Design review of the part built by this model. Coordinates are the model's own, in mm. Face numbers are marked on the shaded views. A direction names the side the tool comes from. Round coordinates to 2 decimals unless told otherwise and drop trailing zeros. Loops run counter-clockwise (first coordinate to the right, second up) from the corner with the lowest first, then second, coordinate; pieces in that order, holes last. Notation, with made-up numbers: M 39,53 L 87,53 A24 ccw 87,82 Z; hole C 0,25.25 d10. An arc over 180 degrees is marked long. One line per item, written item: value. Start each with the question number.
Item 1: Clearance check with a flat-ended pin moving along its axis: pin 1 (1 mm diameter, centred on y = 3, z = -19, fed in from +X). State where the tip first meets the part, or that it passes through.
Item 2: We need section C-C (z = -10.75). Write out the cut boundary in (x, y).
Item 3: For the marked faces 1 and 2, list the 3-axis set-ups (+Z, -Z, +X, -X, +Y, -Y) from which the entire face can be reached by the end or side of a thin tool; tool diameter is ignored.
Item 4: Mouldability with a two-part tool opening along Z and no side actions: class the marked faces 3, 4 and 5 as released by +Z, released by -Z, zero draft, split by the parting line, or undercut.
Item 5: We need section A-A (y = 0.55). Write out the cut boundary in (x, z).
Item 6: We need section B-B (x = -27.5). Write out the cut boundary in (y, z).
Item 7: We need section D-D (x = -29). Write out the cut boundary in (y, z).
Item 8: For line 1 along Z through (x, y) = (-27.75, 1.95); line 2 along Z through (x, y) = (-27.5, 2.1); line 3 along X through (y, z) = (0.45, -19.5), list the stretches that pass through material, from the lowest coordinate up.
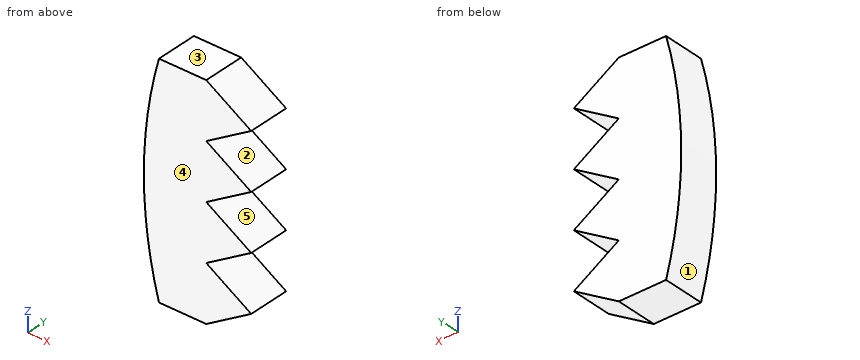
from build123d import *

# Parameters (mm, degrees)
BOSS_EXTRUDE1_DEPTH = 3.81


with BuildPart() as part:
    # Sketch1 → Boss-Extrude1 (new body)
    with BuildSketch(Plane(origin=(0, 0, 0), x_dir=(1, 0, 0), z_dir=(0, 1, 0))):
        with BuildLine():
            Line((-30.793742763, 27.560180372), (-26.69024718, 25.020180372))
            Line((-26.69024718, 25.020180372), (-30.793742763, 22.480180372))
            Line((-30.793742763, 22.480180372), (-26.69024718, 19.940180372))
            Line((-26.69024718, 19.940180372), (-30.793742763, 17.400180372))
            Line((-30.793742763, 17.400180372), (-26.69024718, 14.860180372))
            Line((-26.69024718, 14.860180372), (-30.793742763, 12.320180372))
            Line((-30.793742763, 12.320180372), (-26.69024718, 9.780180372))
            Line((-26.69024718, 9.780180372), (-30.793742763, 7.240180372))
            Line((-30.793742763, 7.240180372), (-35.111742763, 7.240180372))
            ThreePointArc((-35.111742763, 7.240180372), (-36.491388734, 17.400180372), (-35.111742763, 27.560180372))
            Line((-35.111742763, 27.560180372), (-30.793742763, 27.560180372))
        make_face()
    extrude(amount=BOSS_EXTRUDE1_DEPTH)


solid = part.part
A:
1. pin 1: x = -27.4
2. outline: M -35.91,0 L -28.26,0 L -28.26,3.81 L -35.91,3.81 Z
3. face 1: -X, +Y, -Y
3. face 2: +X, +Y, -Y
4. face 3: released by +Z
4. face 4: zero draft
4. face 5: undercut
5. outline: M -35.11,-27.56 L -30.79,-27.56 L -26.69,-25.02 L -30.79,-22.48 L -26.69,-19.94 L -30.79,-17.4 L -26.69,-14.86 L -30.79,-12.32 L -26.69,-9.78 L -30.79,-7.24 L -35.11,-7.24 A38.1 ccw Z
6. outline: M 0,-25.52 L 3.81,-25.52 L 3.81,-24.52 L 0,-24.52 Z; M 0,-20.44 L 3.81,-20.44 L 3.81,-19.44 L 0,-19.44 Z; M 0,-15.36 L 3.81,-15.36 L 3.81,-14.36 L 0,-14.36 Z; M 0,-10.28 L 3.81,-10.28 L 3.81,-9.28 L 0,-9.28 Z
7. outline: M 0,-26.45 L 3.81,-26.45 L 3.81,-23.59 L 0,-23.59 Z; M 0,-21.37 L 3.81,-21.37 L 3.81,-18.51 L 0,-18.51 Z; M 0,-16.29 L 3.81,-16.29 L 3.81,-13.43 L 0,-13.43 Z; M 0,-11.21 L 3.81,-11.21 L 3.81,-8.35 L 0,-8.35 Z
8. line 1: -25.68 to -24.36, -20.6 to -19.28, -15.52 to -14.2, -10.44 to -9.12
8. line 2: -25.52 to -24.52, -20.44 to -19.44, -15.36 to -14.36, -10.28 to -9.28
8. line 3: -36.43 to -27.4
